from build123d import *

# Parameters (mm, degrees)
SKETCH1_R                                      = 20.5
SKETCH1_R_2                                    = 1.5875
SKETCH1_R_3                                    = 13.5
EXTRUDE1_DEPTH                                 = 1.5
BOSS_EXTRUDE3_START                            = -1.5
SKETCH4_R                                      = 23.5
SKETCH4_R_2                                    = 20.5
BOSS_EXTRUDE3_DEPTH                            = 1.5
BOSS_EXTRUDE5_START                            = 21.9577
SKETCH5_R                                      = 23.5
SKETCH5_R_2                                    = 22
BOSS_EXTRUDE5_DEPTH                            = 21.9577
CSK_FOR_0_FLAT_HEAD_MACHINE_SCREW1_D           = 1.6129
CSK_FOR_0_FLAT_HEAD_MACHINE_SCREW1_CSINK_D     = 3.0226
CSK_FOR_0_FLAT_HEAD_MACHINE_SCREW1_CSINK_ANGLE = 82


with BuildPart() as part:
    # Sketch1 → Extrude1 (new body)
    # profile 1 of 4: a face of its own
    with BuildSketch(Plane.XY):
        Circle(SKETCH1_R)
        with Locations((-14.289419162, -8.25)):
            Circle(SKETCH1_R_2, mode=Mode.SUBTRACT)
        with Locations((14.289419162, -8.25)):
            Circle(SKETCH1_R_2, mode=Mode.SUBTRACT)
        with Locations((0, 16.5)):
            Circle(SKETCH1_R_2, mode=Mode.SUBTRACT)
        Circle(SKETCH1_R_3, mode=Mode.SUBTRACT)
    # profile 2 of 4: a face of its own
    with BuildSketch(Plane.XY):
        with Locations((14.289419162, -8.25)):
            Circle(SKETCH1_R_2)
    # profile 3 of 4: a face of its own
    with BuildSketch(Plane.XY):
        with Locations((0, 16.5)):
            Circle(SKETCH1_R_2)
    # profile 4 of 4: a face of its own
    with BuildSketch(Plane.XY):
        with Locations((-14.289419162, -8.25)):
            Circle(SKETCH1_R_2)
    extrude(amount=EXTRUDE1_DEPTH)

    # Sketch4 → Boss-Extrude3 (add)
    with BuildSketch(Plane.XY.offset(1.5).offset(BOSS_EXTRUDE3_START)):
        Circle(SKETCH4_R)
        Circle(SKETCH4_R_2, mode=Mode.SUBTRACT)
    extrude(amount=BOSS_EXTRUDE3_DEPTH)

    # Sketch5 → Boss-Extrude5 (add)
    with BuildSketch(Plane(origin=(0, 0, 0), x_dir=(-1, 0, 0), z_dir=(0, 0, -1)).offset(BOSS_EXTRUDE5_START)):
        with Locations(Location((0, 0, 0), (0, 0, 180))):
            Circle(SKETCH5_R)
        Circle(SKETCH5_R_2, mode=Mode.SUBTRACT)
    extrude(amount=-BOSS_EXTRUDE5_DEPTH)

    # CSK for #0 Flat Head Machine Screw1 (through all)
    with Locations(Plane(origin=(0, 16.5, 1.5), x_dir=(1, 0, 0), z_dir=(0, 0, 1))):
        with Locations((0, 0), (14.289419162, -24.75), (-14.289419162, -24.75)):
            CounterSinkHole(CSK_FOR_0_FLAT_HEAD_MACHINE_SCREW1_D / 2, CSK_FOR_0_FLAT_HEAD_MACHINE_SCREW1_CSINK_D / 2, counter_sink_angle=CSK_FOR_0_FLAT_HEAD_MACHINE_SCREW1_CSINK_ANGLE)


solid = part.part
Source: CAD feature listing. Evaluate the final solid. Frame: model axes, mm. A direction names the side the tool comes from. Give positions to 0.01 mm unless a question says otherwise; leave off trailing zeros. Write each loop counter-clockwise with the first axis right and the second up, starting at its lowest first coordinate (ties: lowest second). Pieces come first, ordered by that corner, then holes. Notation, with made-up numbers: M 63,-9 L 80,-9 A25 ccw 80,27 Z; hole C -25,33.25 d10. An arc over 180 degrees is marked long. Answer as a JSON object with one key per item and string values.
Q1. Cut plane A-A, the plane y = 0. Return the cut outline in (x, z), then the cut area to 3 significant figures.
Geometry check:
{"outline": "M -23.5,-21.96 L -22,-21.96 L -22,0 L -13.5,0 L -13.5,1.5 L -23.5,1.5 Z; M 13.5,0 L 22,0 L 22,-21.96 L 23.5,-21.96 L 23.5,1.5 L 13.5,1.5 Z", "area": "95.9 mm^2"}
Q2. Access query for faces 1 (the face through (9.5, 10.1, 0)), 2 (the face through (0.17, 15.71, 0.34)). Directions: +Z, -Z, +X, -X, +Y, -Y. A direction counts if a zero-diameter tool reaches every point of the face in a straight line with its end or side. Return the directions, or none.
Geometry check:
{"face 1": "-Z", "face 2": "+Z, -Z"}
Q3. Cut plane C-C, the plane y = -8.25. Return the cut outline in (x, z).
Geometry check:
{"outline": "M -22,-21.96 L -20.39,-21.96 L -20.39,0 L -15.1,0 L -15.1,0.69 L -15.8,1.5 L -22,1.5 Z; M -13.48,0 L -10.69,0 L -10.69,1.5 L -12.78,1.5 L -13.48,0.69 Z; M 10.69,0 L 13.48,0 L 13.48,0.69 L 12.78,1.5 L 10.69,1.5 Z; M 15.1,0 L 20.39,0 L 20.39,-21.96 L 22,-21.96 L 22,1.5 L 15.8,1.5 L 15.1,0.69 Z"}
Q4. Contact query for flat-ended pins moving along their axis: P1, Ø12, axis at x = 17, z = -3, coming from the -Y side; P2, Ø1.9, axis at x = 14.29, y = -8.25, coming from the +Z side; P3, Ø2.5, axis at x = 0, y = 16.5, coming from the +Z side. Output: stop coordinate, or through.
Geometry check:
{"P1": "stops at y = -20.77", "P2": "stops at z = 0.85", "P3": "stops at z = 1.2"}
Q5. Ray query, line 1 along Y through (x, z) = (0, 0.5); line 2 along Y through (x, z) = (0.5, -4.5); line 3 along Z through (x, y) = (-13.5, -10). Return the intervals inside material, ascending.
Geometry check:
{"line 1": "y = -23.5 to -13.5, 13.5 to 15.69, 17.31 to 23.5", "line 2": "y = -23.49 to -21.99, 21.99 to 23.49", "line 3": "z = 0 to 1.5"}
Q6. Cut plane D-D, the plane z = -9.25. Return the cut outline in (x, y).
Geometry check:
{"outline": "C 0,0 d47; hole C 0,0 d44"}
Q7. Mould query, pull axis Y, two halves, no side actions, for faces 3 (the face through (16, 16, -21.958)), 4 (the face through (-15.06, -8.01, 0.34)), 5 (the face through (-3.06, -23.3, -10.39)). Classes: +Y half, -Y half, draft (parallel to the pull), parting line (faces both ways), or undercut.
Geometry check:
{"face 3": "draft", "face 4": "undercut", "face 5": "parting line"}
Q8. Cut plane B-B, the plane x = 0. Return the cut outline in (y, z), then the cut area to 3 significant figures.
Geometry check:
{"outline": "M -23.5,-21.96 L -22,-21.96 L -22,0 L -13.5,0 L -13.5,1.5 L -23.5,1.5 Z; M 13.5,0 L 15.69,0 L 15.69,0.69 L 14.99,1.5 L 13.5,1.5 Z; M 17.31,0 L 22,0 L 22,-21.96 L 23.5,-21.96 L 23.5,1.5 L 18.01,1.5 L 17.31,0.69 Z", "area": "92.9 mm^2"}
